```python
from build123d import *

# Parameters (mm, degrees)
BASPROSKE_W      = 10
BASPROSKE_H      = 11
TOOTHCUT_DEPTH   = 19.493242009
TEETHCUTS_COUNT  = 20
TEETHCUTS_ANGLE  = 342
HUBNEAONESKE_R   = 8
HUBNEARONE_DEPTH = 8.0000508
BORSKE_R         = 5
BORE_DEPTH       = 18.0000508


with BuildPart() as part:
    # BasProSke → Base-Revolve (revolve)
    with BuildSketch(Plane(origin=(0, 0, 0), x_dir=(1, 0, 0), z_dir=(0, 1, 0)), mode=Mode.PRIVATE) as base_revolve_sk:
        with Locations((5, 5.5)):
            Rectangle(BASPROSKE_W, BASPROSKE_H)
    revolve(base_revolve_sk.sketch.rotate(Axis((-10, 0, 0), (1, 0, 0)), 180), axis=Axis((-10, 0, 0), (1, 0, 0)))

    # TooCutSke → ToothCut (cut, through all)
    with BuildSketch(Plane(origin=(0, 0, 0), x_dir=(0, 0, -1), z_dir=(1, 0, 0))):
        with BuildLine():
            ThreePointArc((0.499924007, 8.734705318), (0, 8.749), (-0.499924007, 8.734705318))
            ThreePointArc((-0.499924007, 8.734705318), (-0.824302243, 9.905497836), (-1.485192705, 10.924909509))
            ThreePointArc((-1.485192705, 10.924909509), (0, 11.0254), (1.485192705, 10.924909509))
            ThreePointArc((1.485192705, 10.924909509), (0.824302243, 9.905497836), (0.499924007, 8.734705318))
        make_face()
    toothcut = extrude(amount=TOOTHCUT_DEPTH, mode=Mode.SUBTRACT)

    # TeethCuts: ToothCut ×20 about axis
    teethcuts_axis = Axis((-10, 0, 0), (1, 0, 0))
    for i in range(1, TEETHCUTS_COUNT):
        add(toothcut.rotate(teethcuts_axis, i * TEETHCUTS_ANGLE / (TEETHCUTS_COUNT - 1)), mode=Mode.SUBTRACT)

    # HubNeaOneSke → HubNearOne (add)
    with BuildSketch(Plane.ZY):
        with Locations(Location((0, 0, 0), (0, 0, 180))):
            Circle(HUBNEAONESKE_R)
    extrude(amount=HUBNEARONE_DEPTH)

    # BorSke → Bore (cut, symmetric)
    with BuildSketch(Plane(origin=(0, 0, 0), x_dir=(0, 0, -1), z_dir=(1, 0, 0))):
        with Locations(Location((0, 0, 0), (0, 0, 180))):
            Circle(BORSKE_R)
    extrude(amount=BORE_DEPTH, both=True, mode=Mode.SUBTRACT)


solid = part.part
```
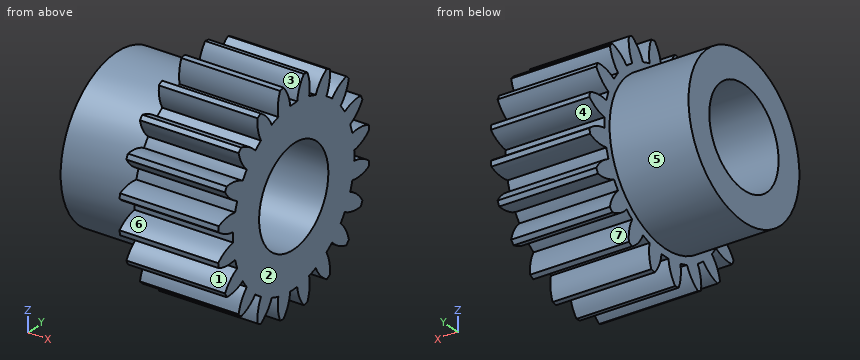
Geometry: final body of the model. Coordinates: model frame, mm. Face numbers are marked on the shaded views. A direction names the side the tool comes from. Round coordinates to 2 decimals unless told otherwise and drop trailing zeros. Order: outer loops, then holes, each group sorted by start corner. A loop starts at its lowest first (then second) coordinate and runs counter-clockwise, first axis right, second up. Notation, with made-up numbers: (-40, -39) - (-13, -39) arc R37 cw to (-13, 0) - close; hole circle Ø10 at (-39, 18.5). An arc over 180 degrees is marked (long way). Use CSV: the item, a comma, the result in double quotes. Start each with the question number.
Q1. Section query D-D (y = 6.25). Return loops of the section in (x, z).
Q2. Section query C-C (z = 6). Return loops of the section in (x, y).
Q3. Mould query, pull axis Z, two halves, no side actions, for the marked faces 1, 2 and 3. Classes: +Z half, -Z half, draft (parallel to the pull), parting line (faces both ways), or undercut.
Q4. First-contact query: pin 1 (1.5 mm diameter, centred on x = -5.5, z = -8, fed in from +Y); pin 2 (1.5 mm diameter, centred on x = 5.5, z = -3.5, fed in from -Y); pin 3 (5 mm diameter, centred on x = -4.5, y = -4.5, fed in from +Z). Flat tips, straight axial feed; report the tip coordinate or a pass-through.
Q5. Material intervals for line 1 along Z through (x, y) = (6.25, 9.75); line 2 along Y through (x, z) = (6, -3.25); line 3 along Y through (x, z) = (-4.25, -2.75), sorted ascending. Write a range as from..to.
Q6. Section query A-A (z = 0). Return loops of the section in (x, y), and give its area (3 significant figures).
Q7. Access query for the marked faces 4, 5, 6 and 7. Directions: +Z, -Z, +X, -X, +Y, -Y. A direction counts if a zero-diameter tool reaches every point of the face in a straight line with its end or side. Return the directions, or none.
Result set:
1,outline,"(-8, -4.99) - (0, -4.99) - (0, -7.38) - (10, -7.38) - (10, 7.38) - (0, 7.38) - (0, 4.99) - (-8, 4.99) - close"
2,outline,"(-8, -5.29) - (0, -5.29) - (0, -7.2) - (10, -7.2) - (10, 7.2) - (0, 7.2) - (0, 5.29) - (-8, 5.29) - close"
3,face 1,"undercut"
3,face 2,"draft"
3,face 3,"+Z half"
4,pin 1,"stops at y = 3.38"
4,pin 2,"stops at y = -9.55"
4,pin 3,"stops at z = 7.75"
5,line 1,"z = -5.09..-4.51, -2.27..-0.76, 0.76..2.27, 4.51..5.09"
5,line 2,"y = -8.31..-3.8, 3.8..8.31"
5,line 3,"y = -7.51..-4.18, 4.18..7.51"
6,outline,"(-8, -8) - (0, -8) - (0, -8.75) - (10, -8.75) - (10, -5) - (-8, -5) - close; (-8, 5) - (10, 5) - (10, 8.75) - (0, 8.75) - (0, 8) - (-8, 8) - close"
6,area,"123 mm2"
7,face 4,"+X, -X, +Y"
7,face 5,"-X"
7,face 6,"+X, -X, -Y"
7,face 7,"+X, -X"
